Source: CAD feature listing. Evaluate the final solid. Frame: model axes, mm. A direction names the side the tool comes from. Coordinates: 2 decimals unless noted, no trailing zeros. Loops run counter-clockwise (first coordinate to the right, second up) from the corner with the lowest first, then second, coordinate; pieces in that order, holes last. Notation, with made-up numbers: M 79.25,19.5 L 133.25,19.5 A28 cw 133.25,50.5 Z; hole C -3.5,14.5 d6. An arc over 180 degrees is marked long. Write each question's results on one line, items separated by ' | '. Start each with the question number.
from build123d import *

# Parameters (mm, degrees)
SKETCH1_W           = 13.3
SKETCH1_H           = 10.5
BOSS_EXTRUDE1_DEPTH = 1.6
SKETCH2_R           = 1.5
CUT_EXTRUDE1_DEPTH  = 1.6
SKETCH3_W           = 2.4
SKETCH3_H           = 4.4
BOSS_EXTRUDE2_DEPTH = 1
FILLET1_R           = 0.5


with BuildPart() as part:
    # Sketch1 → Boss-Extrude1 (new body)
    with BuildSketch(Plane.XY):
        Rectangle(SKETCH1_W, SKETCH1_H)
    extrude(amount=BOSS_EXTRUDE1_DEPTH)

    # Sketch2 → Cut-Extrude1 (cut)
    with BuildSketch(Plane.XY.offset(1.6)):
        with Locations((3.65, 2.25)):
            Circle(SKETCH2_R)
    extrude(amount=-CUT_EXTRUDE1_DEPTH, mode=Mode.SUBTRACT)

    # Sketch3 → Boss-Extrude2 (add)
    with BuildSketch(Plane.XY.offset(1.6)):
        with Locations((2.45, -2.05)):
            Rectangle(SKETCH3_W, SKETCH3_H)
    extrude(amount=BOSS_EXTRUDE2_DEPTH)

    # Fillet1
    fillet1_edges = [part.edges().sort_by_distance(p)[0] for p in [
        (-6.65, 5.25, 0.8),
        (6.65, 5.25, 0.8),
        (6.65, -5.25, 0.8),
        (-6.65, -5.25, 0.8),
    ]]
    fillet(fillet1_edges, radius=FILLET1_R)


solid = part.part
Item 1: First-contact query: pin 1 Ø4 at (x, y) = (-1, -1) entering from +Z. Flat tip, straight axial feed; report the tip coordinate or a pass-through.
Item 2: Cut plane C-C (z = 0.75). Output: boundary loops of the cut face in (x, y).
Item 3: Cut plane D-D (y = -3.5). Output: boundary loops of the cut face in (x, z), then the cut area to 3 significant figures.
Item 4: Line query: probe 1 along Y at (x, z) = (3.65, 1.25); probe 2 along Z at (x, y) = (-1.25, 0.75); probe 3 along X at (y, z) = (-3.5, 2.4). Output: solid intervals per line, ascending.
Item 5: Cut plane A-A (y = 2.25). Output: boundary loops of the cut face in (x, z).
Item 6: Cut plane B-B (x = 2). Output: boundary loops of the cut face in (y, z).
Item 7: Access query for faces 4 (the flat face through (2, 0.15, 2)), 5 (the flat face through (2, -4.25, 2)), 6 (the flat face through (3.65, -2, 2)). Directions: +Z, -Z, +X, -X, +Y, -Y. A direction counts if a zero-diameter tool reaches every point of the face in a straight line with its end or side. Return the directions, or none.
Item 8: Mould query, pull axis X, two halves, no side actions, for faces 1 (the cylindrical face through (3.325, 0.786, 0.811)), 2 (the flat face through (1.25, -2, 2)), 3 (the flat face through (2, -2, 2.6)). Classes: +X half, -X half, draft (parallel to the pull), parting line (faces both ways), or undercut.
Response values:
1) pin 1: stops at z = 1.6
2) outline: M -6.65,-4.75 A0.5 ccw -6.15,-5.25 L 6.15,-5.25 A0.5 ccw 6.65,-4.75 L 6.65,4.75 A0.5 ccw 6.15,5.25 L -6.15,5.25 A0.5 ccw -6.65,4.75 Z; hole C 3.65,2.25 d3
3) outline: M -6.65,0 L 6.65,0 L 6.65,1.6 L 3.65,1.6 L 3.65,2.6 L 1.25,2.6 L 1.25,1.6 L -6.65,1.6 Z | area: 23.7 mm2
4) probe 1: y = -5.25 to 0.75, 3.75 to 5.25 | probe 2: z = 0 to 1.6 | probe 3: x = 1.25 to 3.65
5) outline: M -6.65,0 L 2.15,0 L 2.15,1.6 L -6.65,1.6 Z; M 5.15,0 L 6.65,0 L 6.65,1.6 L 5.15,1.6 Z
6) outline: M -5.25,0 L 5.25,0 L 5.25,1.6 L 0.15,1.6 L 0.15,2.6 L -4.25,2.6 L -4.25,1.6 L -5.25,1.6 Z
7) face 4: +Z, +X, -X, +Y | face 5: +Z, +X, -X, -Y | face 6: +Z, +X, +Y, -Y
8) face 1: undercut | face 2: -X half | face 3: draft
